Answer from the drawing. Dimensions are ordinates in mm from the lowest x, y and z of the part. Give positions to 0.01 mm unless a question says otherwise; leave off trailing zeros. Loops run counter-clockwise (first coordinate to the right, second up) from the corner with the lowest first, then second, coordinate; pieces in that order, holes last. Notation, with made-up numbers: (23.5, 82.25) -> (59.5, 82.25) arc R16 ccw to (59.5, 96.25) -> close; hole circle Ø5 at (24.25, -20.75). An arc over 180 degrees is marked (long way). Write each question's results on one line, items separated by ' | '. Start each with the question number.
Item 1: Section C-C on z = 6.25 is taken. Write down the section's boundary in (x, y), and give its area (3 significant figures).
Item 2: Section A-A on y = 40 is taken. Write down the section's boundary in (x, z), and give its area (3 significant figures).
Item 3: Find the intervals of material crossed by line 1 (Y direction, x = 5, z = 5); line 2 (Y direction, x = 3.5, z = 3.75), in increasing order.
Item 4: This flat-tipped pin is pushed along its axis until it touches: P1, Ø3.5, axis at x = 40, y = 5, coming from the -Z side. Where does it stop, or does it pass through?
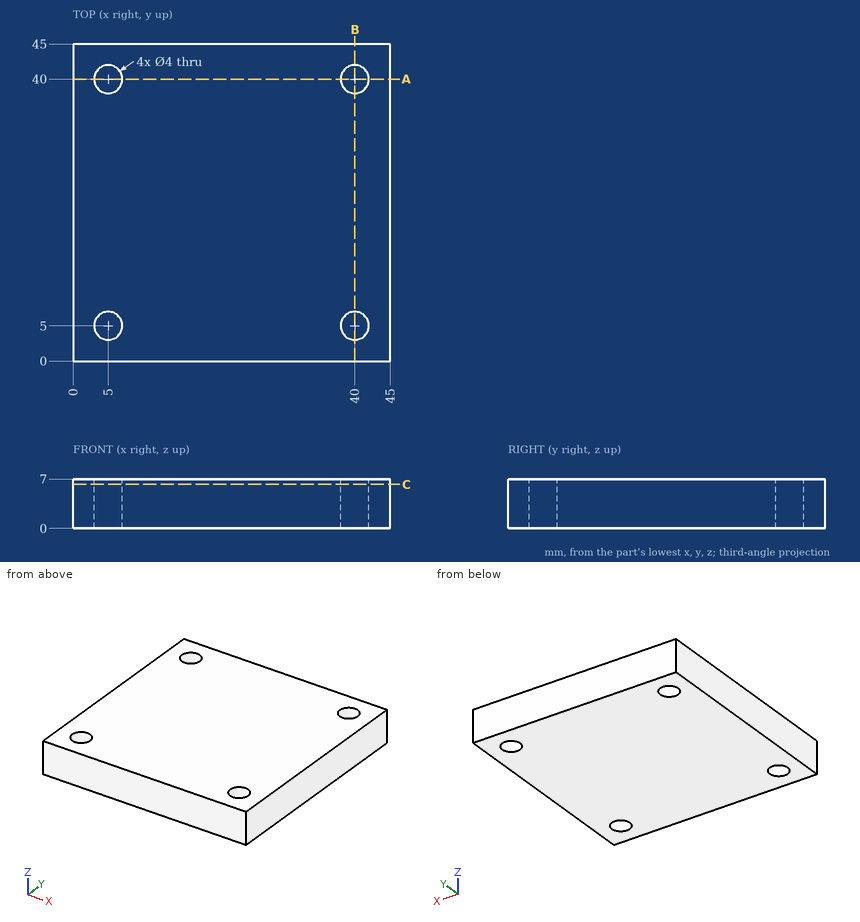
Findings:
1) outline: (0, 0) -> (45, 0) -> (45, 45) -> (0, 45) -> close; hole circle Ø4 at (5, 5); hole circle Ø4 at (5, 40); hole circle Ø4 at (40, 5); hole circle Ø4 at (40, 40) | area: 1,970 mm2
2) outline: (0, 0) -> (3, 0) -> (3, 7) -> (0, 7) -> close; (7, 0) -> (38, 0) -> (38, 7) -> (7, 7) -> close; (42, 0) -> (45, 0) -> (45, 7) -> (42, 7) -> close | area: 259 mm2
3) line 1: 0 to 3, 7 to 38, 42 to 45 | line 2: 0 to 3.68, 6.32 to 38.68, 41.32 to 45
4) P1: through
